Can you work these out from the model? Positions are in its coordinate system, mm. A direction names the side the tool comes from. Give positions to 0.01 mm unless a question says otherwise; leave off trailing zeros. Order: outer loops, then holes, each group sorted by start corner. A loop starts at its lowest first (then second) coordinate and runs counter-clockwise, first axis right, second up.
Item 1: If I drill on line 1 along Y through (x, z) = (43, 1.25); line 2 along Y through (x, z) = (-33.5, 5.75); line 3 along Z through (x, y) = (-40, 80), over which ranges is the centre line in solid material (lowest first)?
Item 2: I want a section at A-A, the plane x = -35.5. Write out the boundary of the cut face in (y, z), then the cut area to 3 significant figures.
Item 3: I'm going to push flat-ended pins straight in: pin 1 Ø1.6 at (x, y) = (89.5, -32) entering from -Z; pin 2 Ø0.6 at (x, y) = (0.5, -92.5) entering from -Z; pin 3 Ø2.5 at (y, z) = (43, 6) entering from -X. Where does each tip first touch, or does it pass through?
Item 4: I want a section at B-B, the plane y = 83. Write out the boundary of the cut face in (x, z), then the cut area to 3 significant figures.
Item 5: If we mould it in two halves opening along Y, with no side actions, what happens to faces 1 (the flat face through (0.8, 95.263, 7.2)), 2 (the flat face through (-82.885, -46.965, 7.249)), 3 (the flat face through (-56, 88, 0)), 4 (the flat face through (0, -45.033, 7))? For each: +Y half, -Y half, draft (parallel to the pull), parting line (faces both ways), or undercut.
Item 6: I want a section at C-C, the plane x = -96. Write out the boundary of the cut face in (y, z), then the cut area to 3 significant figures.
Item 7: Which directions (+Z, -Z, +X, -X, +Y, -Y) give clear straight access to the entire face, cutting with the end or side of a thin tool? Please do faces 5 (the flat face through (-79.87, 45.26, 7.15)), 6 (the flat face through (85, -39, 0)).
```python
from build123d import *

# Parameters (mm, degrees)
PAD_DEPTH       = 12
POCKET_DEPTH    = 4
POCKET001_DEPTH = 2
POCKET002_DEPTH = 3.2
POCKET003_DEPTH = 5
POCKET004_DEPTH = 8
SKETCH007_W     = 6
SKETCH007_H     = 7
POCKET005_DEPTH = 2
SKETCH008_W     = 5
SKETCH008_H     = 6
SKETCH008_H_2   = 5.175393
POCKET006_DEPTH = 7
SKETCH009_W     = 10
SKETCH009_H     = 4
PAD001_DEPTH    = 3
POCKET007_DEPTH = 52


with BuildPart() as part:
    # Sketch → Pad (new body)
    with BuildSketch(Plane.XY):
        Polygon((-110, 0), (-55, -95.262794), (55, -95.262794), (110, 0), (55, 95.262794), (-55, 95.262794), align=None)
    extrude(amount=PAD_DEPTH)

    # Sketch001 (on Face8 of Pad) → Pocket (cut)
    with BuildSketch(Plane.XY.offset(12)):
        Polygon((-50.1, 0), (-25.05, -43.387873), (25.05, -43.387873), (50.1, 0), (25.05, 43.387873), (-25.05, 43.387873), align=None)
    extrude(amount=-POCKET_DEPTH, mode=Mode.SUBTRACT)

    # Sketch002 (on Face4 of Pocket) → Pocket001 (cut)
    with BuildSketch(Plane(origin=(0, 0, 0), x_dir=(1, 0, 0), z_dir=(0, 0, -1))):
        with BuildLine():
            Line((-106, 0), (-53, -91.798693))
            Line((53, -91.798693), (-53, -91.798693))
            Line((53, -91.798693), (106, 0))
            Line((53, 91.798693), (106, 0))
            Line((1.5, 91.798693), (53, 91.798693))
            Line((1.5, 91.798693), (1.5, 92.298693))
            ThreePointArc((1.5, 92.298693), (0, 93.798693), (-1.5, 92.298693))
            Line((-1.5, 91.798693), (-1.5, 92.298693))
            Line((-53, 91.798693), (-1.5, 91.798693))
            Line((-106, 0), (-53, 91.798693))
        make_face()
    extrude(amount=-POCKET001_DEPTH, mode=Mode.SUBTRACT)

    # Sketch003 (on Face26 of Pocket001) → Pocket002 (cut)
    with BuildSketch(Plane.XY.offset(8)):
        Polygon((-48.615, 0), (-24, -42.351379), (-12.5, -42.351379), (-12.5, -44.351379), (12.5, -44.351379), (12.5, -42.351379), (24, -42.351379), (48.615, 0), (25.5, 39.770552), (23.8, 39.770552), (23.8, 44.21), (14.6, 44.21), (14.6, 41.41), (4.4, 41.41), (4.4, 44.21), (-4.8, 44.21), (-4.8, 41.41), (-14.2, 41.41), (-14.2, 44.21), (-23.4, 44.21), (-23.4, 39.770552), (-25.5, 39.770552), align=None)
    extrude(amount=-POCKET002_DEPTH, mode=Mode.SUBTRACT)

    # Sketch005 (on Face56 of Pocket002) → Pocket003 (cut)
    with BuildSketch(Plane.XY.offset(4.8)):
        Polygon((-24, -41.569219), (24, -41.569219), (48, 0), (27.792741, 35), (-27.792741, 35), (-48, 0), align=None)
    extrude(amount=-POCKET003_DEPTH, mode=Mode.SUBTRACT)

    # Sketch006 (on Face25 of Pocket003) → Pocket004 (cut)
    with BuildSketch(Plane(origin=(0, 0, 2), x_dir=(1, 0, 0), z_dir=(0, 0, -1))):
        Polygon((106, 0), (53, 91.798693), (-53, 91.798693), (-106, 0), (-53, -91.798693), (53, -91.798693), align=None)
        Polygon((-26.5, -43.8), (26.5, -43.8), (52, 0), (26, 45.033321), (-26, 45.033321), (-52, 0), align=None, mode=Mode.SUBTRACT)
    extrude(amount=-POCKET004_DEPTH, mode=Mode.SUBTRACT)

    # Sketch007 (on Face14 of Pocket004) → Pocket005 (cut)
    with BuildSketch(Plane(origin=(0, -91.798693, 0), x_dir=(-1, 0, 0), z_dir=(0, 1, 0))):
        with Locations((0, 5.5)):
            Rectangle(SKETCH007_W, SKETCH007_H)
    extrude(amount=-POCKET005_DEPTH, mode=Mode.SUBTRACT)

    # Sketch008 (on Face4 of Pocket005) → Pocket006 (cut)
    with BuildSketch(Plane(origin=(0, 0, 0), x_dir=(1, 0, 0), z_dir=(0, 0, -1))):
        with Locations((-17.5, -93.155396)):
            Rectangle(SKETCH008_W, SKETCH008_H)
        with Locations((17.5, -93.155396)):
            Rectangle(SKETCH008_W, SKETCH008_H)
        with Locations((-17.5, 92.844604)):
            Rectangle(SKETCH008_W, SKETCH008_H)
        with Locations((17.5, 92.844604)):
            Rectangle(SKETCH008_W, SKETCH008_H)
        Polygon((72.943614, -65.208026), (67.747462, -62.208026), (70.247462, -57.877899), (75.443614, -60.877899), align=None)
        Polygon((91.08198, -35.276307), (85.885827, -32.276307), (88.385827, -27.94618), (93.58198, -30.94618), align=None)
        Polygon((-88.307892, 27.495521), (-93.504045, 30.495521), (-90.832982, 35.121938), (-85.636829, 32.121938), align=None)
        Polygon((-70.637333, 58.102991), (-75.833485, 61.102991), (-73.162422, 65.729408), (-67.96627, 62.729408), align=None)
        Polygon((68.025973, 62.368825), (73.222126, 65.368825), (75.722126, 61.038698), (70.525973, 58.038698), align=None)
        Polygon((85.525973, 32.057936), (90.722126, 35.057936), (93.222126, 30.727809), (88.025973, 27.727809), align=None)
        Polygon((-93.477396, -30.875189), (-88.281244, -27.875189), (-85.781244, -32.205316), (-90.977396, -35.205316), align=None)
        Polygon((-75.942627, -61.165973), (-70.746474, -58.165973), (-68.246474, -62.4961), (-73.442627, -65.4961), align=None)
        with Locations((0, -93.5677)):
            Rectangle(SKETCH008_W, SKETCH008_H_2)
        Polygon((-85.225594, -46.318269), (-80.029442, -43.318269), (-77.529442, -47.648396), (-82.725594, -50.648396), align=None)
        Polygon((76.42707, 47.011941), (81.623222, 50.011941), (84.123222, 45.681814), (78.92707, 42.681814), align=None)
        Polygon((-79.184311, 42.830332), (-84.380464, 45.830332), (-81.880464, 50.160459), (-76.684311, 47.160459), align=None)
        Polygon((82.868303, -50.730789), (77.672151, -47.730789), (80.172151, -43.400661), (85.368303, -46.400661), align=None)
    extrude(amount=-POCKET006_DEPTH, mode=Mode.SUBTRACT)

    # Sketch009 (on Face116 of Pocket006) → Pad001 (join)
    with BuildSketch(Plane.XZ.offset(45.033321)):
        with Locations((-21, 4)):
            Rectangle(SKETCH009_W, SKETCH009_H)
        with Locations((21, 4)):
            Rectangle(SKETCH009_W, SKETCH009_H)
    extrude(amount=PAD001_DEPTH)

    # Sketch010 (on Face155 of Pad001) → Pocket007 (cut)
    with BuildSketch(Plane(origin=(-26, 0, 0), x_dir=(0, -1, 0), z_dir=(-1, 0, 0))):
        Polygon((45.049209, 6.011785), (48.049209, 2.011785), (48.049209, 6.011785), align=None)
    extrude(amount=-POCKET007_DEPTH, mode=Mode.SUBTRACT)


solid = part.part
```
Results list:
1. line 1: y = -95.26 to -91.8, 91.8 to 95.26
1. line 2: y = -95.26 to -91.8, -32.04 to -26.01, 26.01 to 31.78, 91.8 to 95.26
1. line 3: z = 10 to 12
2. outline: (-95.26, 0) - (-91.8, 0) - (-91.8, 10) - (-28.58, 10) - (-28.58, 2) - (-21.65, 2) - (-21.65, 4.8) - (-22.57, 4.8) - (-22.57, 8) - (-25.29, 8) - (-25.29, 12) - (-95.26, 12) - close; (21.65, 2) - (28.34, 2) - (28.34, 10) - (91.8, 10) - (91.8, 0) - (95.26, 0) - (95.26, 12) - (25.29, 12) - (25.29, 8) - (22.57, 8) - (22.57, 4.8) - (21.65, 4.8) - close
2. area: 438 mm2
3. pin 1: stops at z = 7
3. pin 2: stops at z = 9
3. pin 3: stops at x = -85.9
4. outline: (-62.08, 0) - (-58.08, 0) - (-58.08, 10) - (58.08, 10) - (58.08, 0) - (62.08, 0) - (62.08, 12) - (-62.08, 12) - close
4. area: 328 mm2
5. face 1: +Y half
5. face 2: -Y half
5. face 3: draft
5. face 4: undercut
6. outline: (-24.25, 0) - (-17.32, 0) - (-17.32, 10) - (17.32, 10) - (17.32, 0) - (24.25, 0) - (24.25, 12) - (-24.25, 12) - close
6. area: 236 mm2
7. face 5: -Z
7. face 6: -Z, +X, -X, +Y, -Y
